Geometry: final body of the model. Coordinates: model frame, mm. Round coordinates to 2 decimals unless told otherwise and drop trailing zeros. Loops run counter-clockwise (first coordinate to the right, second up) from the corner with the lowest first, then second, coordinate; pieces in that order, holes last. Notation, with made-up numbers: (-3.75, 52.25) - (17.25, 52.25) arc R18 cw to (17.25, 69.25) - close; hole circle Ø8 at (78.25, 79.25). An arc over 180 degrees is marked (long way). Answer as a JSON object with one key per item and string values. Group by question number.
Item 1: Section A-A (z = 0.1). Return the cut outline in (x, y).
Item 2: Line query: line 1 (X direction, y = 3.75, z = 0.1); line 2 (X direction, y = 6.25, z = -0.3); line 3 (X direction, y = 1, z = 0.3). Output: solid intervals per line, ascending.
Item 3: First-contact query: pin 1 (2 mm diameter, centred on x = 19.5, y = 4.5, fed in from -Z). Flat tip, straight axial feed; report the tip coordinate or a pass-through.
Item 4: Draft query along Y for faces 1 (the face through (1.214, 9.375, -0.011)), 2 (the face through (0, 5, 0)), 3 (the face through (11, 10.185, 0)). Return one class per face: released by +Y, released by -Y, zero draft, split by the parting line, or undercut.
```python
from build123d import *

# Parameters (mm, degrees)
SKETCH1_W           = 22.917169521
SKETCH1_H           = 10.185584258
SKETCH1_R           = 1.509847023
SKETCH1_R_2         = 0.476625594
BOSS_EXTRUDE1_DEPTH = 0.81


with BuildPart() as part:
    # Sketch1 → Boss-Extrude1 (new, symmetric)
    with BuildSketch(Plane.XY):
        with Locations((11.45856993, 5.092103028)):
            Rectangle(SKETCH1_W, SKETCH1_H)
        with Locations((20.383783826, 5.092103028)):
            Circle(SKETCH1_R, mode=Mode.SUBTRACT)
        with Locations((1.27648108, 8.902103028)):
            Circle(SKETCH1_R_2, mode=Mode.SUBTRACT)
        with Locations((1.27648108, 6.362103028)):
            Circle(SKETCH1_R_2, mode=Mode.SUBTRACT)
        with Locations((1.27648108, 3.822103028)):
            Circle(SKETCH1_R_2, mode=Mode.SUBTRACT)
        with Locations((1.27648108, 1.282103028)):
            Circle(SKETCH1_R_2, mode=Mode.SUBTRACT)
    extrude(amount=BOSS_EXTRUDE1_DEPTH, both=True)


solid = part.part
```
Values:
{
 "1": {"outline": "(0, 0) - (22.92, 0) - (22.92, 10.18) - (0, 10.18) - close; hole circle Ø0.95 at (1.28, 1.28); hole circle Ø0.95 at (1.28, 3.82); hole circle Ø0.95 at (1.28, 6.36); hole circle Ø0.95 at (1.28, 8.9); hole circle Ø3.02 at (20.38, 5.09)"},
 "2": {"line 1": "x = 0 to 0.81, 1.75 to 19.69, 21.08 to 22.92", "line 2": "x = 0 to 0.81, 1.74 to 19.41, 21.35 to 22.92", "line 3": "x = 0 to 0.89, 1.66 to 22.92"},
 "3": {"pin 1": "stops at z = -0.81"},
 "4": {"face 1": "undercut", "face 2": "zero draft", "face 3": "released by +Y"}
}
